Part model, mm, in its own coordinate system. Round coordinates to 2 decimals unless told otherwise and drop trailing zeros. Order: outer loops, then holes, each group sorted by start corner. A loop starts at its lowest first (then second) coordinate and runs counter-clockwise, first axis right, second up. Notation, with made-up numbers: M 32.5,-3 L 74.5,-3 A9 ccw 74.5,13 Z; hole C 60.25,-25.75 d10. An arc over 180 degrees is marked long. One line per question, with ' | ' between items.
from build123d import *

# Parameters (mm, degrees)
CROQUIS1_W              = 235
CROQUIS1_H              = 35
CROQUIS1_R              = 13.25
CROQUIS1_R_2            = 3.5
SALIENTE_EXTRUIR1_DEPTH = 10
REDONDEO1_R             = 17.5
REDONDEO2_R             = 2


with BuildPart() as part:
    # Croquis1 → Saliente-Extruir1 (new body)
    with BuildSketch(Plane(origin=(0, 0, 0), x_dir=(1, 0, 0), z_dir=(0, 1, 0))):
        with Locations((-117.5, 17.5)):
            Rectangle(CROQUIS1_W, CROQUIS1_H)
        with Locations(Location((-20, 17.5, 0), (0, 0, 270))):
            Circle(CROQUIS1_R, mode=Mode.SUBTRACT)
        with Locations(Location((-220, 17.5, 0), (0, 0, 270))):
            Circle(CROQUIS1_R_2, mode=Mode.SUBTRACT)
    extrude(amount=SALIENTE_EXTRUIR1_DEPTH)

    # Redondeo1
    redondeo1_edges = [part.edges().sort_by_distance(p)[0] for p in [
        (0, 5, 0),
        (0, 5, -35),
        (-235, 5, -35),
        (-235, 5, 0),
    ]]
    fillet(redondeo1_edges, radius=REDONDEO1_R - 0.0001)  # a hair under: the kernel refuses the full size

    # Redondeo2
    redondeo2_edges = [part.edges().sort_by_distance(p)[0] for p in [
        (-117.5, 0, 0),
        (-117.5, 0, -35),
        (-229.87439796, 0, -5.12560204),
        (-229.87439796, 0, -29.87439796),
        (-5.12560204, 0, -29.87439796),
        (-5.12560204, 0, -5.12560204),
        (-117.5, 10, 0),
        (-117.5, 10, -35),
        (-229.87439796, 10, -5.12560204),
        (-229.87439796, 10, -29.87439796),
        (-5.12560204, 10, -29.87439796),
        (-5.12560204, 10, -5.12560204),
    ]]
    fillet(redondeo2_edges, radius=REDONDEO2_R)


solid = part.part
1) Saw through at B-B (y = 6). Give the number of separate pieces and of enclosed holes in the cut face, plus the area to 3 significant figures.
The answers:
separate pieces: 1 | enclosed holes: 2 | area: 7,370 mm²
2) Probe line 1 (X direction, y = 6, z = -17.5); line 2 (X direction, y = 7.5, z = -16); line 3 (X direction, y = 5, z = -13). List the from-to ranges inside material, lowest first. Write a range as [from, to].
The answers:
line 1: x = [-235, -223.5], [-216.5, -33.25], [-6.75, 0] | line 2: x = [-234.94, -223.16], [-216.84, -33.16], [-6.84, -0.06] | line 3: x = [-234.41, -32.46], [-7.54, -0.59]
3) Saw through at A-A (x = -20). List the corners of the cut face in (y, z).
The answers:
outline: M 0,-33 A2 ccw 2,-35 L 8,-35 A2 ccw 10,-33 L 10,-30.75 L 0,-30.75 Z; M 0,-4.25 L 10,-4.25 L 10,-2 A2 ccw 8,0 L 2,0 A2 ccw 0,-2 Z
4) Two-plate mould, pull along Z, no slides. Class faces 1 (the face through (-119, 0, -18)), 2 (the face through (-230.01, 5.04, -29.74)), 3 (the face through (-216.53, 4.93, -17.96)): released by +Z, released by -Z, zero draft, split by the parting line, or undercut.
The answers:
face 1: zero draft | face 2: released by -Z | face 3: undercut
5) Drop flat-ended pins along their axis: pin 1 (1 mm diameter, centred on y = 7.5, z = -19.5, fed in from -X); pin 2 (5.5 mm diameter, centred on x = -220, z = -17.5, fed in from +Y). Give the stop position or say it passes through.
The answers:
pin 1: stops at x = -234.94 | pin 2: passes through
